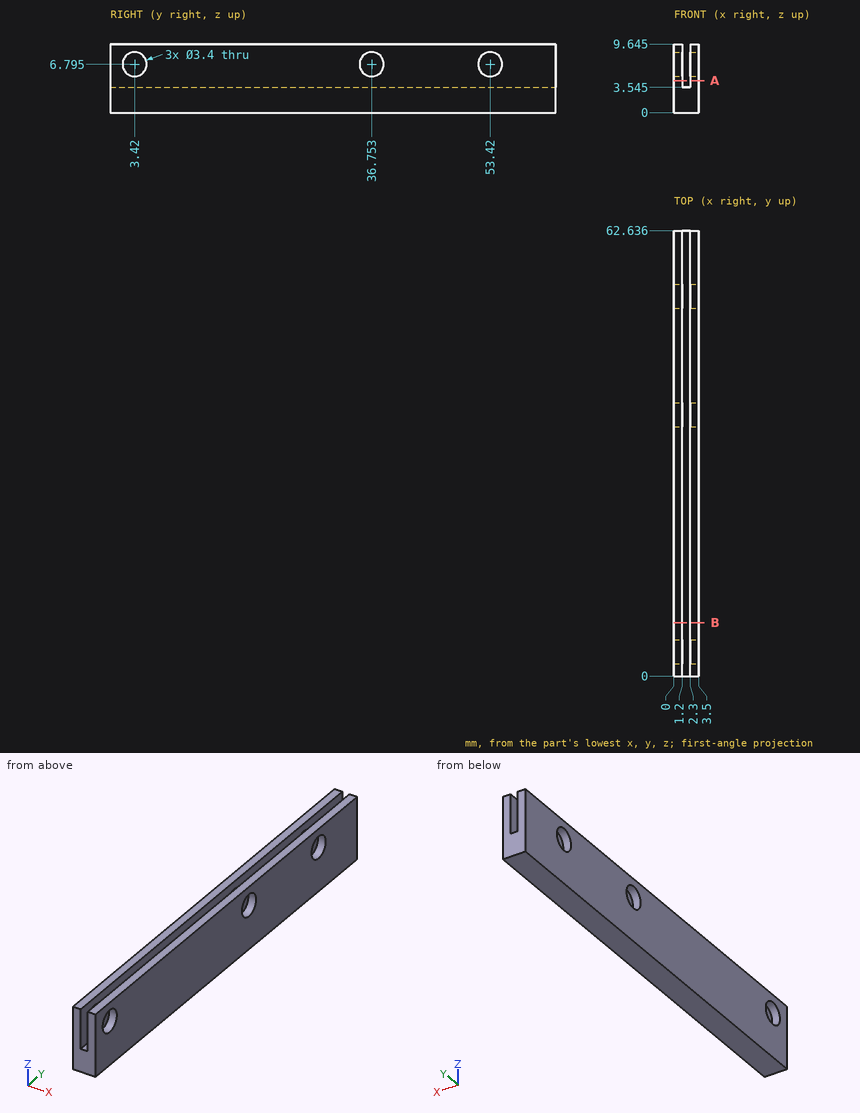
Could you check a few things on this drawing? It's one solid part, dimensions in mm from its lowest x, y, z. Coordinates: 2 decimals unless noted, no trailing zeros. Write each loop counter-clockwise with the first axis right and the second up, starting at its lowest first coordinate (ties: lowest second). Pieces come first, ordered by that corner, then holes. Notation, with made-up numbers: (28.25, 5.25) - (48.25, 5.25) arc R22 cw to (48.25, 25.25) - close; hole circle Ø6 at (-36.75, -7). An arc over 180 degrees is marked (long way). Write item = value, one per line.
1) Suppose I cut it at B-B on y = 7.5. Please give me the cut outline in (x, z) (1 decimal).
Result set:
outline = (0, 0) - (3.5, 0) - (3.5, 9.6) - (2.3, 9.6) - (2.3, 3.5) - (1.2, 3.5) - (1.2, 9.6) - (0, 9.6) - close
2) Please list where these lines run through material, in increasing order: line 1 (X direction, y = 29, z = 6.75); line 2 (Z direction, x = 2.2, y = 20) (1 decimal); line 3 (Z direction, x = 0.6, y = 3) (1 decimal). Write a range as [from, to].
Result set:
line_1 = [0, 1.2], [2.3, 3.5]
line_2 = [0, 3.5]
line_3 = [0, 5.1], [8.4, 9.6]
3) Will this pin go through, and if not, where does the flat tip stop? pin 1 Ø2.5 at (y, z) = (3.42, 6.8) entering from +X.
Result set:
pin_1 = through
4) Suppose I cut it at A-A on z = 4.5. Please give me the cut outline in (x, y).
Result set:
outline = (0, 0) - (1.2, 0) - (1.2, 62.64) - (0, 62.64) - close; (2.3, 0) - (3.5, 0) - (3.5, 62.64) - (2.3, 62.64) - close
